Part model, mm, in its own coordinate system. A direction names the side the tool comes from. Round coordinates to 2 decimals unless told otherwise and drop trailing zeros. Write each loop counter-clockwise with the first axis right and the second up, starting at its lowest first coordinate (ties: lowest second). Pieces come first, ordered by that corner, then holes. Notation, with made-up numbers: (64.5, 26) -> (68.5, 26) arc R16 cw to (68.5, 51) -> close; hole circle Ø8 at (3, -2). An arc over 180 degrees is marked (long way). Return JSON: item names as keys, results as strings. Group by question number.
(1) Drill centre lines: L1, parallel to Z at x = -2.25, y = 1.25 (3 decimals); L2, parallel to Y at x = 0, z = 5.75; L3, parallel to X at y = -1.5, z = 3. Where is each one in solid material? Low to high. Write a range as from..to.
(2) Saw through at A-A (y = 0). List the corners of the cut face in (x, z) (3 decimals), plus the area to 3 significant figures.
(3) Tool access for faces 1 (the cylindrical face through (-3, 0, 2)), 2 (the flat face through (0, 0, -0.25)): list every direction of +Z, -Z, +X, -X, +Y, -Y with a clear straight run to the whole face (end or side of a thin tool).
(4) Saw through at D-D (z = 2.75). List the corners of the cut face in (x, y), plus the area to 3 significant figures.
(5) Saw through at C-C (z = 5.5). List the corners of the cut face in (x, y), plus the area to 3 significant figures.
(6) Drop flat-ended pins along their axis: pin 1 Ø1.5 at (x, y) = (-5, 3) entering from +Z; pin 2 Ø1.5 at (y, z) = (-1.5, 2) entering from +X; pin 3 Ø3 at (y, z) = (5, 0.5) entering from +X. Give the stop position or say it passes through.
from build123d import *

# Parameters (mm, degrees)
F0_R     = 2.5
F1_DEPTH = 3.375
F0_R_2   = 3
F2_DEPTH = 1.375
F0_R_3   = 6.5
F3_DEPTH = 0.875
F4_DEPTH = 0.25
F7_DEPTH = 2.76
F8_DEPTH = 2.76
F9_SIZE  = 0.25


with BuildPart() as f1:
    # F0 (on Top) → F1 (new body)
    with BuildSketch(Plane.XY):
        Circle(F0_R)
    extrude(amount=F1_DEPTH)

    # F0 (on Top) → F2 (join)
    with BuildSketch(Plane.XY):
        Circle(F0_R_2)
        Circle(F0_R, mode=Mode.SUBTRACT)
    extrude(amount=F2_DEPTH)

    # F0 (on Top) → F3 (join)
    with BuildSketch(Plane.XY):
        Circle(F0_R_3)
        Circle(F0_R_2, mode=Mode.SUBTRACT)
    extrude(amount=F3_DEPTH)

    # F0 (on Top) → F4 (join)
    with BuildSketch(Plane.XY):
        Circle(F0_R_3)
        Circle(F0_R_2, mode=Mode.SUBTRACT)
        Circle(F0_R_2)
        Circle(F0_R, mode=Mode.SUBTRACT)
        Circle(F0_R)
    extrude(amount=-F4_DEPTH)

    # F5 (on Right) → F6 (revolve, cut)
    with BuildSketch(Plane.YZ):
        Polygon((-6.6943974234, 0.9619678603), (-6.6943974234, 0), (-3.1168663409, 0.9619678603), align=None)
    revolve(axis=Axis((0, 0, 0.9346584557), (0, 0, 1)), mode=Mode.SUBTRACT)

    # F7 (add): a face of the model
    f7_faces = [f1.faces().sort_by_distance(p)[0] for p in [
        (-2.9151471863, 0, 1.375),
    ]]
    extrude(f7_faces, amount=F7_DEPTH)

    # F8 (add): a face of the model
    f8_faces = [f1.faces().sort_by_distance(p)[0] for p in [
        (0, 0, 3.375),
    ]]
    extrude(f8_faces, amount=F8_DEPTH)

    # F9
    f9_edges = [f1.edges().sort_by_distance(p)[0] for p in [
        (-2.5, 0, 6.135),
    ]]
    chamfer(f9_edges, length=F9_SIZE)


solid = f1.part
Computed values:
{
 "1": {"L1": "-0.25..4.135", "L2": "-2.5..2.5", "L3": "-2.6..2.6"},
 "2": {"outline": "(-6.5, -0.25) -> (6.5, -0.25) -> (6.5, 0.052) -> (3.44, 0.875) -> (3, 0.875) -> (3, 4.135) -> (2.5, 4.135) -> (2.5, 5.885) -> (2.25, 6.135) -> (-2.25, 6.135) -> (-2.5, 5.885) -> (-2.5, 4.135) -> (-3, 4.135) -> (-3, 0.875) -> (-3.44, 0.875) -> (-6.5, 0.052) -> close", "area": "41.6 mm2"},
 "3": {"face 1": "+Z", "face 2": "-Z, +X, -X, +Y, -Y"},
 "4": {"outline": "circle Ø6 at (0, 0)", "area": "28.3 mm2"},
 "5": {"outline": "circle Ø5 at (0, 0)", "area": "19.6 mm2"},
 "6": {"pin 1": "z = 0.43", "pin 2": "x = 2.9", "pin 3": "x = 5.43"}
}
